Autodesk Inventor part; units mm, degrees
ref_plane "YZ Plane" through (0, 0, 0) normal (1, 0, 0) x (0, 1, 0)
ref_plane "XZ Plane" through (0, 0, 0) normal (0, 1, 0) x (-1, 0, 0)
ref_plane "XY Plane" through (0, 0, 0) normal (0, 0, 1) x (1, 0, 0)
sketch "Skizze1" plane through (0, 0, 0) normal (0, 1, 0) x (-1, 0, 0)
  circle A0 centre (0, 0) radius 4
  circle A1 centre (0, 0) radius 1.25
  line L0 (0, -4) -> (0, 21.2)
  line L1 (0, 21.2) -> (0, 18.9)
  circle A2 centre (0, 18.9) radius 0.6
  circle A3 centre (0, 18.9) radius 2.3
  line L2 (0, 18.9) -> (0, 16.1)
  line L3 (0, 16.1) -> (0, 13.3)
  circle A4 centre (0, 16.1) radius 0.6
  line L4 (0, 16.1) -> (0, 13.3)
  circle A5 centre (0, 13.3) radius 0.6
  line L5 (0, 13.3) -> (0, 10.5)
  circle A6 centre (0, 10.5) radius 0.6
  line L6 (0, 10.5) -> (0, 7.7)
  circle A7 centre (0, 7.7) radius 0.6
  line L7 (0, 7.7) -> (0, 4.9)
  circle A8 centre (0, 4.9) radius 0.6
  circle A9 centre (0, 10.5) radius 0.75
  line L8 (0.75, 10.5) -> (2.2, 3.3407)
  line L9 (-0.75, 10.5) -> (-2.2, 3.3407)
  circle A10 centre (0, 0) radius 2.95
  circle A11 centre (0, 0) radius 2.55
  line L10 (-3.7997, 1.25) -> (-2.3, 18.9)
  line L11 (3.7997, 1.25) -> (2.3, 18.9)
  point P0 (-4, 0)
  point P1 (4, 0)
  point P2 (0.3, 16.6196)
  point P3 (-0.3, 16.6196)
  dimension "d0" = 8
  dimension "d2" = 2.5
  dimension "d4" = 25.2
  dimension "d5" = 2.3
  dimension "d6" = 1.2
  dimension "d7" = 2.8
  dimension "d10" = 1.2
  dimension "d11" = 2.8
  dimension "d12" = 1.2
  dimension "d13" = 2.8
  dimension "d14" = 1.2
  dimension "d15" = 2.8
  dimension "d16" = 1.2
  dimension "d17" = 2.8
  dimension "d18" = 1.2
  dimension "d19" = 1.5
  dimension "d20" = 5.9
  dimension "d21" = 5.1
extrude "Extrusion1" add sketch "Skizze1" along normal blind 1.6 contours A0 L0 A10 | A0 L8 A9 L0 A5 A4 A3 L11 | A0 L0 A10 | A0 L0 A8 A7 A9 L8 | A3 A4 L0 A2 | L10 A3 A4 L0 A5 A9 L9 A0 | A10 L0 A11 | L0 A11 A10 | A0 L9 A9 L0 A7 A8 | A9 L0 A6 | L0 A2 A4 A3 | L0 A6 A9
extrude "Extrusion2" add sketch "Skizze1" along normal blind 2.8 contours A0 L0 A10 | A0 L0 A10 | A0 L0 A8 A7 A9 L8 | A10 L0 A11 | L0 A11 A10 | A0 L9 A9 L0 A7 A8 | A9 L0 A6 | L0 A6 A9
extrude "Extrusion3" add sketch "Skizze1" along normal blind 4.1 contours A0 L0 A10 | A0 L0 A10 | A10 L0 A11 | L0 A11 A10
extrude "Extrusion4" add sketch "Skizze1" along normal blind 1 contours A11 L0 A1 | L0 A1 A11
extrude "Extrusion5" cut sketch "Skizze1" along normal blind 0.5 contours A10 L0 A11 | L0 A11 A10 | A11 L0 A1 | L0 A1 A11
properties part number "weißes_ding" material "Plastic, Opaque White"
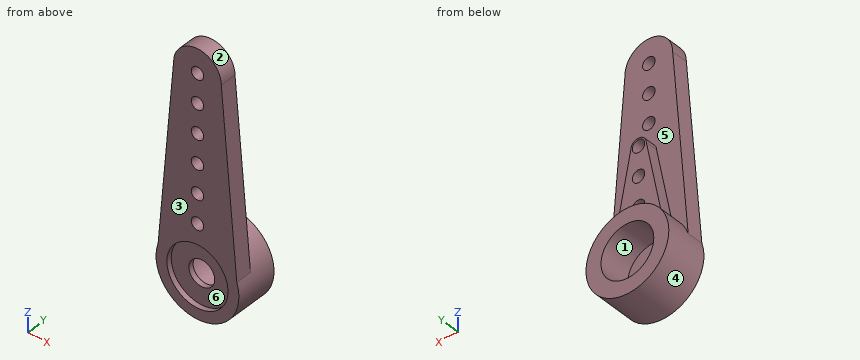
Source: CAD feature listing. Evaluate the final solid. Frame: model axes, mm. Face numbers are marked on the shaded views. A direction names the side the tool comes from. Give positions to 0.01 mm unless a question says otherwise; leave off trailing zeros. Write each loop counter-clockwise with the first axis right and the second up, starting at its lowest first coordinate (ties: lowest second). Pieces come first, ordered by that corner, then holes. Notation, with made-up numbers: (31.5, 5) - (60.5, 5) arc R36 ccw to (60.5, 43) - close; hole circle Ø6 at (34, 7.5). An arc over 180 degrees is marked (long way). One line per item, written item: value. Start each with the question number.
Q1. Draft query along Z for the marked faces 1, 2 and 3. Return one class per face: +Z half, -Z half, draft (parallel to the pull), parting line (faces both ways), or undercut.
Q2. Material intervals for probe 1 along Z at (x, y) = (0, 3.5); probe 2 along X at (y, z) = (2.6, 10.5); probe 3 along Y at (x, z) = (0, 15), sorted ascending. Write a range as from..to.
Q3. First-contact query: pin 1 Ø4 at (x, z) = (0, 12.5) entering from +Y; pin 2 Ø0.7 at (x, z) = (0, 16.1) entering from -Y; pin 3 Ø4.5 at (x, z) = (0.5, 0) entering from -Y. Flat tips, straight axial feed; report the tip coordinate or a pass-through.
Q4. Set-up query: the marked faces 4, 5 and 6. Return all of +Z, -Z, +X, -X, +Y, -Y with unobstructed straight access to the full face (end or side cutting, diameter ignored); none if empty.
Q5. Section query C-C, the plane x = -0.25. Count the separate pieces of the cut face and the enclosed holes in it, then the cut area to 3 significant figures.
Q6. Section query A-A, the plane z = 13.3. Return the cut outline in (x, y), then the cut area to 3 significant figures.
Q7. Section query D-D, the plane x = 1.5. Return the cut outline in (y, z), then the cut area to 3 significant figures.
Q8. Section query B-B, the plane y = 1.3. Return the cut outline in (x, z), then the cut area to 3 significant figures.
Answer:
1. face 1: undercut
1. face 2: +Z half
1. face 3: draft
2. probe 1: z = -4..-2.55, 2.55..4
2. probe 2: x = -0.75..-0.6, 0.6..0.75
2. probe 3: y = 0..1.6
3. pin 1: stops at y = 2.8
3. pin 2: passes through
3. pin 3: stops at y = 0.5
4. face 4: +Y
4. face 5: +Z, +Y
4. face 6: -Y
5. separate pieces: 8
5. enclosed holes: 0
5. area: 34.6 mm2
6. outline: (-2.78, 0) - (-0.6, 0) - (-0.6, 1.6) - (-2.78, 1.6) - close; (0.6, 0) - (2.78, 0) - (2.78, 1.6) - (0.6, 1.6) - close
6. area: 6.96 mm2
7. outline: (0, -3.71) - (4.1, -3.71) - (4.1, -2.06) - (1, -2.06) - (1, 2.06) - (4.1, 2.06) - (4.1, 3.71) - (2.8, 3.71) - (2.8, 6.8) - (1.6, 6.8) - (1.6, 20.64) - (0, 20.64) - (0, 2.54) - (0.5, 2.54) - (0.5, -2.54) - (0, -2.54) - close
7. area: 45.9 mm2
8. outline: (-3.8, 1.25) arc R4 ccw (long way) to (3.8, 1.25) - (2.3, 18.9) arc R2.3 ccw to (-2.3, 18.9) - close; hole circle Ø5.1 at (0, 0); hole circle Ø1.2 at (0, 4.9); hole circle Ø1.2 at (0, 7.7); hole circle Ø1.2 at (0, 10.5); hole circle Ø1.2 at (0, 13.3); hole circle Ø1.2 at (0, 16.1); hole circle Ø1.2 at (0, 18.9)
8. area: 124 mm2
